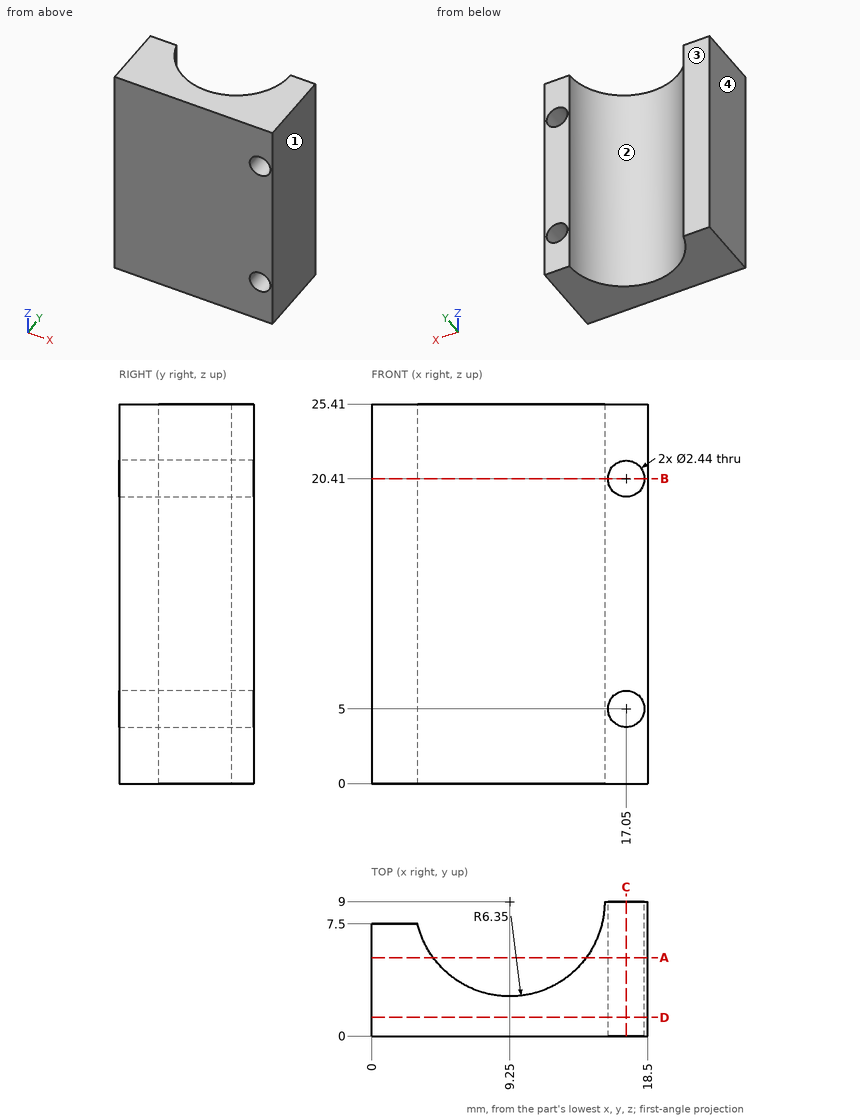
Here's the drawing with two shaded views (mm, measured from the low corner). I have some questions. Round coordinates to 2 decimals unless told otherwise and drop trailing zeros. Write each loop counter-clockwise with the first axis right and the second up, starting at its lowest first coordinate (ties: lowest second). Pieces come first, ordered by that corner, then holes.
(1) Thinking about a two-plate mould opening in X: for the marked faces 1, 2, 3 and 4, which applies, +X half, -X half, draft (parallel to the pull), parting line (faces both ways), or undercut?
Findings below:
face 1: +X half
face 2: undercut
face 3: draft
face 4: -X half
(2) Suppose I cut it at D-D on y = 1.25. Write out the boundary of the cut face in (x, z).
Findings below:
outline: (0, 0) - (18.5, 0) - (18.5, 25.41) - (0, 25.41) - close; hole circle Ø2.44 at (17.05, 5); hole circle Ø2.44 at (17.05, 20.41)
(3) Suppose I cut it at A-A on y = 5.25. Write out the boundary of the cut face in (x, z), and give its area (3 significant figures).
Findings below:
outline: (0, 0) - (4.13, 0) - (4.13, 25.41) - (0, 25.41) - close; (14.37, 0) - (18.5, 0) - (18.5, 25.41) - (14.37, 25.41) - close; hole circle Ø2.44 at (17.05, 5); hole circle Ø2.44 at (17.05, 20.41)
area: 200 mm2
(4) Suppose I cut it at C-C on x = 17.05. Write out the boundary of the cut face in (y, z).
Findings below:
outline: (0, 0) - (9, 0) - (9, 3.78) - (0, 3.78) - close; (0, 6.22) - (9, 6.22) - (9, 19.19) - (0, 19.19) - close; (0, 21.63) - (9, 21.63) - (9, 25.41) - (0, 25.41) - close
(5) Suppose I cut it at B-B on z = 20.41. Write out the boundary of the cut face in (x, y), and give its area (3 significant figures).
Findings below:
outline: (0, 0) - (15.83, 0) - (15.83, 9) - (15.6, 9) arc R6.35 cw to (3.08, 7.5) - (0, 7.5) - close; (18.27, 0) - (18.5, 0) - (18.5, 9) - (18.27, 9) - close
area: 76.8 mm2
(6) For pin 1 (1.5 mm diameter, centred on x = 1, z = 15.5, fed in from +Y), with a flat end and sliding along its axis, tell me the tip position at first contact or that it passes through.
Findings below:
pin 1: stops at y = 7.5
(7) If I drill on probe 1 along X at (y, z) = (3.75, 20.41); probe 2 along Y at (x, z) = (1.5, 17); probe 3 along X at (y, z) = (7.25, 23), over which ranges is the centre line in solid material (lowest first)?
Findings below:
probe 1: x = 0 to 5.68, 12.82 to 15.83, 18.27 to 18.5
probe 2: y = 0 to 7.5
probe 3: x = 0 to 3.15, 15.35 to 18.5
